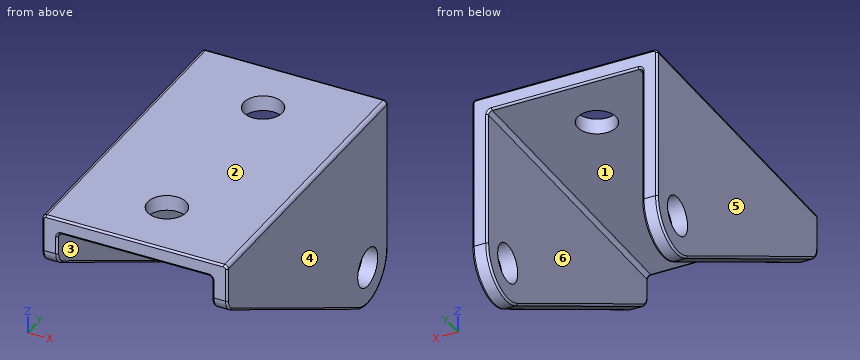
```python
from build123d import *

# Parameters (mm, degrees)
BOSS_EXTRUDE1_DEPTH = 40
SKETCH2_OUTSIDE_W   = 37.584
SKETCH2_OUTSIDE_H   = 52.584
CUT_EXTRUDE1_DEPTH  = 30
FILLET1_R           = 0.25
SKETCH3_R           = 2.5
CUT_EXTRUDE2_DEPTH  = 40
SKETCH4_R           = 2.5
CUT_EXTRUDE3_DEPTH  = 30


with BuildPart() as part:
    # Sketch1 → Boss-Extrude1 (new body)
    with BuildSketch(Plane(origin=(0, 0, 0), x_dir=(1, 0, 0), z_dir=(0, 1, 0))):
        with BuildLine():
            Line((12, -1.5), (12, 23))
            Line((12, 23), (10, 23))
            Line((10, 23), (10, 0.5))
            ThreePointArc((10, 0.5), (9.853553391, 0.146446609), (9.5, 0))
            Line((9.5, 0), (-9.5, 0))
            ThreePointArc((-9.5, 0), (-9.853553391, 0.146446609), (-10, 0.5))
            Line((-10, 0.5), (-10, 23))
            Line((-10, 23), (-12, 23))
            Line((-12, 23), (-12, -1.5))
            ThreePointArc((-12, -1.5), (-11.853553391, -1.853553391), (-11.5, -2))
            Line((-11.5, -2), (11.5, -2))
            ThreePointArc((11.5, -2), (11.853553391, -1.853553391), (12, -1.5))
        make_face()
    extrude(amount=BOSS_EXTRUDE1_DEPTH)

    # Sketch2 outside → Cut-Extrude1 (cut)
    with BuildSketch(Plane.ZY.offset(12)):
        with Locations((-10.5, 20)):
            Rectangle(SKETCH2_OUTSIDE_W, SKETCH2_OUTSIDE_H)
        with BuildLine():
            Line((-22.35505953, 32.543690474), (-4.573869643, 1.017476189))
            ThreePointArc((-4.573869643, 1.017476189), (-3.840546078, 0.273001502), (-2.831845831, 0))
            Line((-2.831845831, 0), (2, 0))
            Line((2, 0), (2, 40))
            Line((2, 40), (-18, 40))
            ThreePointArc((-18, 40), (-22.317496244, 37.521750619), (-22.35505953, 32.543690474))
        make_face(mode=Mode.SUBTRACT)
    extrude(amount=-CUT_EXTRUDE1_DEPTH, mode=Mode.SUBTRACT)

    # Fillet1
    fillet1_edges = [part.edges().sort_by_distance(p)[0] for p in [
        (-10, 0, -1.665922915),
        (-9.853553391, 0, -0.146446609),
        (-11.853553391, 40, 1.853553391),
        (0, 0, 0),
        (9.853553391, 0, -0.146446609),
        (12, 0, -0.665922915),
        (11.853553391, 0, 1.853553391),
        (0, 0, 2),
        (-11.853553391, 0, 1.853553391),
        (0, 40, 2),
        (11.853553391, 40, 1.853553391),
        (12, 40, -8.25),
        (10, 0, -1.665922915),
        (9.853553391, 40, -0.146446609),
        (-12, 0, -0.665922915),
        (-12, 40, -8.25),
        (10, 40, -9.25),
        (0, 40, 0),
        (-10, 16.780583332, -13.464464586),
        (-9.853553391, 40, -0.146446609),
        (-10, 40, -9.25),
        (12, 16.780583332, -13.464464586),
        (-12, 16.780583332, -13.464464586),
        (-12, 37.521750619, -22.317496244),
        (12, 37.521750619, -22.317496244),
        (12, 0.273001502, -3.840546078),
        (-12, 0.273001502, -3.840546078),
        (10, 37.521750619, -22.317496244),
        (-10, 37.521750619, -22.317496244),
        (10, 0.273001502, -3.840546078),
        (-10, 0.273001502, -3.840546078),
        (10, 16.780583332, -13.464464586),
    ]]
    fillet(fillet1_edges, radius=FILLET1_R)

    # Sketch3 → Cut-Extrude2 (cut)
    with BuildSketch(Plane.ZY.offset(12)):
        with Locations((-18, 35)):
            Circle(SKETCH3_R)
    extrude(amount=-CUT_EXTRUDE2_DEPTH, mode=Mode.SUBTRACT)

    # Sketch4 → Cut-Extrude3 (cut)
    with BuildSketch(Plane(origin=(0, 0, 0), x_dir=(-1, 0, 0), z_dir=(0, 0, -1))):
        with Locations((0, 32)):
            Circle(SKETCH4_R)
        with Locations((0, 8)):
            Circle(SKETCH4_R)
    extrude(amount=-CUT_EXTRUDE3_DEPTH, mode=Mode.SUBTRACT)


solid = part.part
```
Here's how the part is built. I have some questions about the finished solid (model axes, mm). Face numbers are marked on the shaded views. A direction names the side the tool comes from. Give positions to 0.01 mm unless a question says otherwise; leave off trailing zeros. Loops run counter-clockwise (first coordinate to the right, second up) from the corner with the lowest first, then second, coordinate; pieces in that order, holes last. Notation, with made-up numbers: M 36.25,40.5 L 85.25,40.5 A24 cw 85.25,58.5 Z; hole C 68,9 d5. An arc over 180 degrees is marked long. Use one line per item in the form item = value. Start each with the question number.
Q1. Thinking about a two-plate mould opening in X: for the marked faces 1, 2, 3 and 4, which applies, +X half, -X half, draft (parallel to the pull), parting line (faces both ways), or undercut?
Q2. If we section it at B-B (y = 35): State how many separate pieces and enclosed holes the cut face has, then the cut area to 3 significant figures.
Q3. Which directions (+Z, -Z, +X, -X, +Y, -Y) give clear straight access to the entire face, cutting with the end or side of a thin tool? Please do the marked faces 5 and 6.
Q4. If we section it at C-C (x = 6): Write out the boundary of the cut face in (y, z), then the cut area to 3 significant figures.
Q5. Will these pins go through, and if not, where does the flat tip stop? pin 1 Ø9.5 at (x, y) = (4, 24.5) entering from -Z; pin 2 Ø4.5 at (x, y) = (0, 32) entering from -Z.
Q6. I need wall thicknesses on line 1 along Y through (x, z) = (0, 0.5); line 2 along X through (y, z) = (30.5, -7.5); line 3 along Z through (x, y) = (0, 38). Which ranges of each line are inside material? Lowest first, please.
Q7. If we section it at A-A (x = 0): Write out the boundary of the cut face in (y, z), then the cut area to 3 significant figures.
Taken from the geometry:
q1.face_1 = undercut
q1.face_2 = draft
q1.face_3 = undercut
q1.face_4 = +X half
q2.separate_pieces = 3
q2.enclosed_holes = 0
q2.area = 120 mm^2
q3.face_5 = +Z, -Z, -X, +Y, -Y
q3.face_6 = -Z, +Y, -Y
q4.outline = M 0,0.25 A0.25 ccw 0.25,0 L 39.75,0 A0.25 ccw 40,0.25 L 40,1.75 A0.25 ccw 39.75,2 L 0.25,2 A0.25 ccw 0,1.75 Z
q4.area = 79.9 mm^2
q5.pin_1 = 0
q5.pin_2 = through
q6.line_1 = 0 to 5.5, 10.5 to 29.5, 34.5 to 40
q6.line_2 = -12 to -10, 10 to 12
q6.line_3 = 0 to 2
q7.outline = M 0,0.25 A0.25 ccw 0.25,0 L 5.5,0 L 5.5,2 L 0.25,2 A0.25 ccw 0,1.75 Z; M 10.5,0 L 29.5,0 L 29.5,2 L 10.5,2 Z; M 34.5,0 L 39.75,0 A0.25 ccw 40,0.25 L 40,1.75 A0.25 ccw 39.75,2 L 34.5,2 Z
q7.area = 59.9 mm^2
